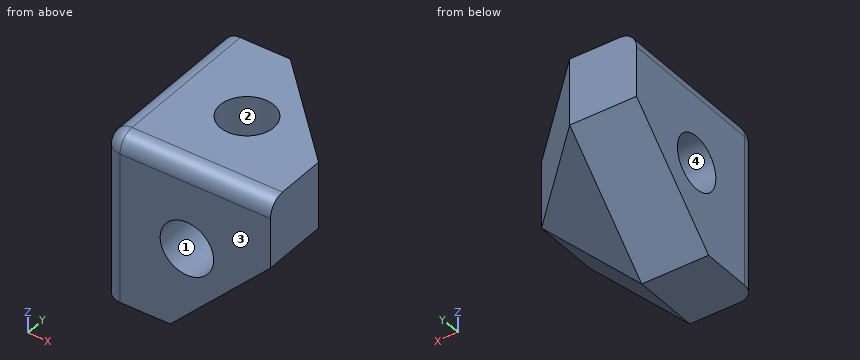
from build123d import *

# Parameters (mm, degrees)
SKETCH1_W           = 10
SKETCH1_H           = 10
BOSS_EXTRUDE1_DEPTH = 10
SKETCH2_R           = 1.6
CUT_EXTRUDE1_DEPTH  = 3.2
SKETCH3_R           = 1.6
CUT_EXTRUDE3_DEPTH  = 3.2
SKETCH4_R           = 1.6
CUT_EXTRUDE4_DEPTH  = 3.2
FILLET2_R           = 1
CHAMFER1_SIZE       = 6


with BuildPart() as part:
    # Sketch1 → Boss-Extrude1 (new body)
    with BuildSketch(Plane(origin=(0, 0, 0), x_dir=(1, 0, 0), z_dir=(0, 1, 0))):
        Rectangle(SKETCH1_W, SKETCH1_H)
    extrude(amount=BOSS_EXTRUDE1_DEPTH)

    # Sketch2 → Cut-Extrude1 (cut)
    with BuildSketch(Plane.XY.offset(5)):
        with Locations((0, 5)):
            Circle(SKETCH2_R)
    extrude(amount=-CUT_EXTRUDE1_DEPTH, mode=Mode.SUBTRACT)

    # Sketch3 → Cut-Extrude3 (cut)
    with BuildSketch(Plane(origin=(0, 0, 0), x_dir=(-1, 0, 0), z_dir=(0, -1, 0))):
        with Locations(Location((0, 0, 0), (0, 0, 90))):
            Circle(SKETCH3_R)
    extrude(amount=-CUT_EXTRUDE3_DEPTH, mode=Mode.SUBTRACT)

    # Sketch4 → Cut-Extrude4 (cut)
    with BuildSketch(Plane(origin=(-5, 0, 0), x_dir=(0, 0, -1), z_dir=(1, 0, 0))):
        with Locations((0, 5)):
            Circle(SKETCH4_R)
    extrude(amount=CUT_EXTRUDE4_DEPTH, mode=Mode.SUBTRACT)

    # Fillet2
    fillet2_edges = [part.edges().sort_by_distance(p)[0] for p in [
        (0, 0, 5),
        (-5, 0, 0),
        (-5, 5, 5),
    ]]
    fillet(fillet2_edges, radius=FILLET2_R)

    # Chamfer1
    chamfer1_edges = [part.edges().sort_by_distance(p)[0] for p in [
        (5, 10, 0),
        (5, 5, -5),
        (0, 10, -5),
    ]]
    chamfer(chamfer1_edges, length=CHAMFER1_SIZE)


solid = part.part
Geometry check sheet. Reference: the model listing, model coordinates, mm. Face numbers are marked on the shaded views. Give positions to 0.01 mm unless a question says otherwise; leave off trailing zeros. Loops run counter-clockwise (first coordinate to the right, second up) from the corner with the lowest first, then second, coordinate; pieces in that order, holes last. Notation, with made-up numbers: (31.5, 77.25) -> (75.5, 77.25) arc R16 ccw to (75.5, 108.25) -> close; hole circle Ø4 at (-37.5, 84.5). An arc over 180 degrees is marked (long way). Answer in a Markdown table with one row per item. Add a question column.
1) Cross-section at C-C on z = 0. Record the boundary of the cut face in (x, y), and give its area (3 significant figures).
2) Draft check along Y on the marked faces 1, 2, 3 and 4. Enter one of: pulls with the +Y half, pulls with the -Y half, needs draft (parallel to the pull), parting line crosses it, or undercut.
3) Gauge pin test, flat ends, axial feed: P1, Ø1.9, axis at x = 0, z = 0, coming from the +Y side; P2, Ø3, axis at y = 5, z = 0, coming from the -X side. Record the tip position at first contact, or that the pin passes through.
4) Material ranges on probe 1 along X at (y, z) = (2, 1.25); probe 2 along X at (y, z) = (2.3, 0); probe 3 along Z at (x, y) = (-2.25, 5.75), recorded low to high. Write a range as from..to.
5) Cross-section at D-D on y = 9.25. Record the boundary of the cut face in (x, z).
6) Cross-section at B-B on y = 1.5. Record the boundary of the cut face in (x, z).
7) Cross-section at A-A on x = -3.5. Record the boundary of the cut face in (y, z).
Outcome:
| question | item | result |
|---|---|---|
| 1 | outline | (-5, 1) arc R1 ccw to (-4, 0) -> (-1.6, 0) -> (-1.6, 3.2) -> (1.6, 3.2) -> (1.6, 0) -> (4, 0) -> (4, 4) -> (-1, 9) -> (-5, 9) -> (-5, 6.6) -> (-1.8, 6.6) -> (-1.8, 3.4) -> (-5, 3.4) -> close |
| 1 | area | 47.8 mm^2 |
| 2 | face 1 | needs draft |
| 2 | face 2 | undercut |
| 2 | face 3 | pulls with the -Y half |
| 2 | face 4 | undercut |
| 3 | P1 | stops at y = 9.34 |
| 3 | P2 | stops at x = -1.8 |
| 4 | probe 1 | x = -5..-1, 1..5 |
| 4 | probe 2 | x = -5..-1.6, 1.6..4 |
| 4 | probe 3 | z = -3.25..-1.41, 1.41..5 |
| 5 | outline | (-5, 0.25) -> (-1, 0.25) -> (-0.25, 1) -> (-0.25, 5) -> (-4, 5) arc R1 ccw to (-5, 4) -> close |
| 6 | outline | (-5, -5) -> (-1, -5) -> (5, 1) -> (5, 5) -> (-4, 5) arc R1 ccw to (-5, 4) -> close; hole circle Ø3.2 at (0, 0) |
| 7 | outline | (0, -5) -> (4, -5) -> (10, 1) -> (10, 5) -> (1, 5) arc R1 ccw to (0, 4) -> close; hole circle Ø3.2 at (5, 0) |
